Can you work these out from the drawing? Everything is in mm from the part's minimum corner. A direction names the side the tool comes from. Coordinates: 2 decimals unless noted, no trailing zeros. Order: outer loops, then holes, each group sorted by start corner. A loop starts at its lowest first (then second) coordinate and runs counter-clockwise, first axis right, second up. Notation, with made-up numbers: M -39,53 L -17,53 A25 cw -17,86 Z; hole C -39,-31.5 d5. An arc over 180 degrees is marked long. Answer as a JSON object with one key per item and string values.
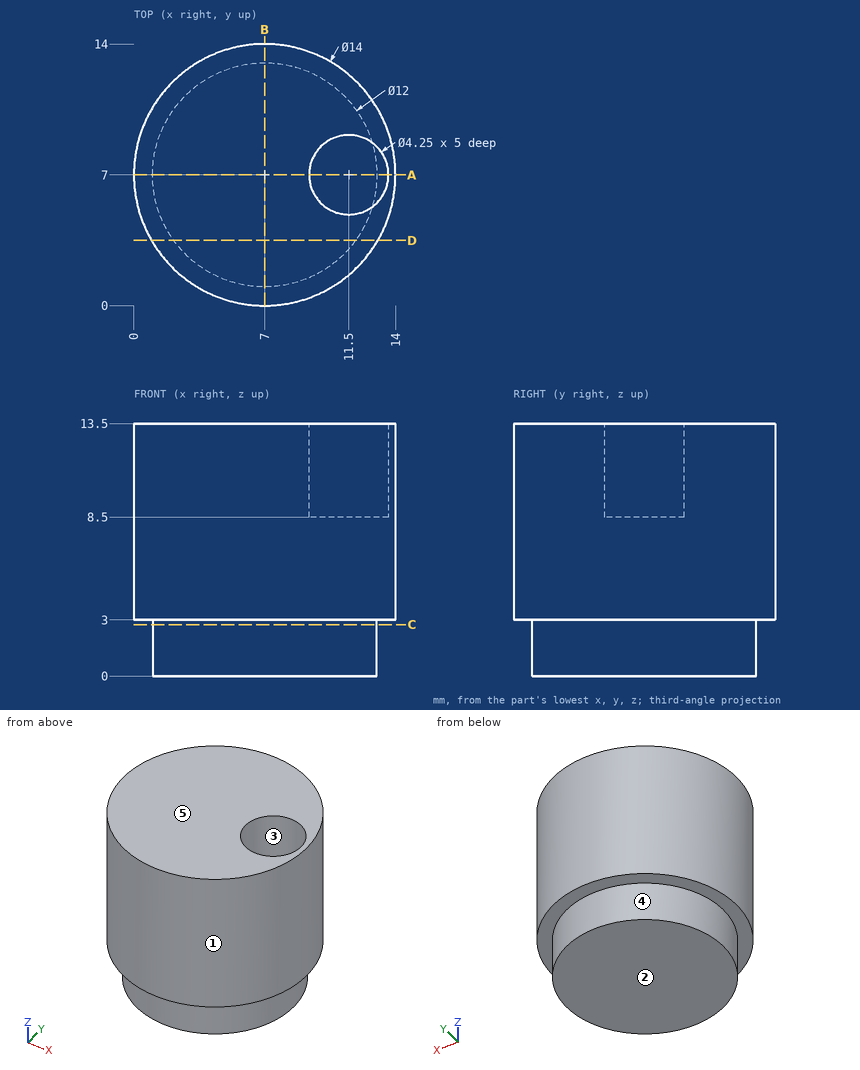
Item 1: If we mould it in two halves opening along X, with no side actions, what happens to the marked faces 1, 2 and 3? For each: pulls with the +X half, pulls with the -X half, needs draft (parallel to the pull), parting line crosses it, or undercut.
Answers follow:
{"face 1": "parting line crosses it", "face 2": "needs draft", "face 3": "undercut"}
Item 2: I want a section at C-C, the plane z = 2.75. Write out the boundary of the cut face in (x, y), plus the area to 3 significant figures.
Answers follow:
{"outline": "C 7,7 d12", "area": "113 mm^2"}
Item 3: Which directions (+Z, -Z, +X, -X, +Y, -Y) give clear straight access to the entire face, cutting with the end or side of a thin tool? Please do the marked faces 4 and 5.
Answers follow:
{"face 4": "-Z", "face 5": "+Z, +X, -X, +Y, -Y"}
Item 4: I want a section at B-B, the plane x = 7. Write out the boundary of the cut face in (y, z).
Answers follow:
{"outline": "M 0,3 L 1,3 L 1,0 L 13,0 L 13,3 L 14,3 L 14,13.5 L 0,13.5 Z"}
Item 5: I want a section at D-D, the plane y = 3.5. Write out the boundary of the cut face in (x, z).
Answers follow:
{"outline": "M 0.94,3 L 2.13,3 L 2.13,0 L 11.87,0 L 11.87,3 L 13.06,3 L 13.06,13.5 L 0.94,13.5 Z"}
Item 6: I want a section at A-A, the plane y = 7. Write out the boundary of the cut face in (x, z) (3 decimals).
Answers follow:
{"outline": "M 0,3 L 1,3 L 1,0 L 13,0 L 13,3 L 14,3 L 14,13.5 L 13.625,13.5 L 13.625,8.5 L 9.375,8.5 L 9.375,13.5 L 0,13.5 Z"}
Item 7: I'm going to push flat-ended pins straight in: pin 1 (4.5 mm diameter, centred on x = 11.5, y = 7, fed in from +Z); pin 2 (3 mm diameter, centred on x = 2.5, z = 9.5, fed in from +Y); pin 3 (3 mm diameter, centred on x = 5, z = 8.5, fed in from -Y); pin 4 (6 mm diameter, centred on y = 10.5, z = 8, fed in from -X). Where does each tip first touch, or does it pass through?
Answers follow:
{"pin 1": "stops at z = 13.5", "pin 2": "stops at y = 13.32", "pin 3": "stops at y = 0.02", "pin 4": "stops at x = 0.02"}
Item 8: Please list where these lines run through material, in increasing order: line 1 (Y direction, x = 11.5, z = 11.7) (3 decimals); line 2 (Y direction, x = 11.25, z = 11); line 3 (Z direction, x = 1.75, y = 2.5).
Answers follow:
{"line 1": "y = 1.638 to 4.875, 9.125 to 12.362", "line 2": "y = 1.44 to 4.89, 9.11 to 12.56", "line 3": "z = 3 to 13.5"}
